The model under review builds one solid part; all positions refer to its coordinate system, in mm. A direction names the side the tool comes from. Coordinates: 2 decimals unless noted, no trailing zeros. Loops run counter-clockwise (first coordinate to the right, second up) from the corner with the lowest first, then second, coordinate; pieces in that order, holes last. Notation, with made-up numbers: (61.5, 70) - (83.5, 70) arc R15 ccw to (83.5, 74) - close; hole circle Ø9 at (63.25, 49). An arc over 180 degrees is marked (long way). Answer in a Markdown table with one row per item. Add a question column.
(1) We need section C-C on z = -5.25. Write out the cut boundary in (x, y), plus the area to 3 significant figures.
(2) We need section B-B on x = 0. Write out the cut boundary in (y, z), plus the area to 3 significant figures.
(3) Machinability: for faces 4 (the cylindrical face through (0.01, 55.65, -0.06)), 5 (the cylindrical face through (-0.867, 40.744, -4.93)), 6 (the flat face through (1, 48, -10)), which of the approach directions +Z, -Z, +X, -X, +Y, -Y give a long, thin tool a straight path to every point of the face, cutting with its end or side? Answer none if there is none.
(4) We need section A-A on y = 60.25. Write out the cut boundary in (x, z).
(5) For P1, Ø6, axis at y = 55.5, z = -4, coming from the -X side; P2, Ø2, axis at y = 52.5, z = -3, coming from the -X side; P3, Ø4, axis at y = 60.5, z = -0.5, coming from the +X side; P4, Ø3.5, axis at x = 0, y = 44.65, coming from the -Z side, all flat-tipped, find the tip position at first contact; note any pin that passes through.
(6) For line 1 along Y through (x, z) = (0, -6.3); line 2 along Y through (x, z) = (0.5, -6.75); line 3 along X through (y, z) = (62.25, -2.5), list the stretches that pass through material, from the lowest coordinate up.
(7) Mouldability with a two-part tool opening along X and no side actions: class faces 1 (the cylindrical face through (0.65, 41.72, -7.54)), 2 (the flat face through (2, 63.649, 0)), 3 (the cylindrical face through (0, 54, 4)) as +X half, -X half, draft (parallel to the pull), parting line (faces both ways), or undercut.
(8) We need section D-D on y = 51.25. Write out the cut boundary in (x, z).
from build123d import *

# Parameters (mm, degrees)
CROQUIS1_R              = 4
SALIENTE_EXTRUIR1_DEPTH = 10
CROQUIS3_R              = 3
CORTAR_EXTRUIR2_DEPTH   = 5
CROQUIS4_W              = 4
CROQUIS4_H              = 19
CROQUIS5_W              = 2
CROQUIS5_H              = 8


with BuildPart() as part:
    # Croquis1 → Saliente-Extruir1 (new body)
    with BuildSketch(Plane.XY):
        with Locations((0, 44.649122807)):
            Circle(CROQUIS1_R)
    extrude(amount=-SALIENTE_EXTRUIR1_DEPTH)

    # Croquis3 → Cortar-Extruir2 (cut)
    with BuildSketch(Plane(origin=(0, 0, -10), x_dir=(-1, 0, 0), z_dir=(0, 0, -1))):
        with Locations((0, 44.649122807)):
            Circle(CROQUIS3_R)
    extrude(amount=-CORTAR_EXTRUIR2_DEPTH, mode=Mode.SUBTRACT)

    # Croquis4 → Revolución1 (revolve)
    with BuildSketch(Plane(origin=(0, 0, 0), x_dir=(0, 0, -1), z_dir=(1, 0, 0)), mode=Mode.PRIVATE) as revoluci_n1_sk:
        with Locations((-2, 54.149122807)):
            Rectangle(CROQUIS4_W, CROQUIS4_H)
    revolve(revoluci_n1_sk.sketch.rotate(Axis((0, 44.649122807, 0), (0, 1, 0)), 180), axis=Axis((0, 44.649122807, 0), (0, 1, 0)))

    # Croquis5 → Cortar-Revolución1 (revolve, cut)
    with BuildSketch(Plane(origin=(0, 63.649122807, 0), x_dir=(1, 0, 0), z_dir=(0, 1, 0))):
        with Locations((0, 4)):
            Rectangle(CROQUIS5_W, CROQUIS5_H)
    revolve(axis=Axis((1, 63.649122807, 0), (-1, 0, 0)), mode=Mode.SUBTRACT)

    # Croquis6 → Revolución3 (revolve)
    with BuildSketch(Plane.XZ.offset(-44.649122807)):
        with BuildLine():
            Line((-4, 0), (4, 0))
            ThreePointArc((4, 0), (0, 4), (-4, 0))
        make_face()
    revolve(axis=Axis((-4, 44.649122807, 0), (1, 0, 0)))


solid = part.part
Outcome:
| question | item | result |
|---|---|---|
| 1 | outline | circle Ø8 at (0, 44.65); hole circle Ø6 at (0, 44.65) |
| 1 | area | 22.0 mm² |
| 2 | outline | (40.65, -10) - (41.65, -10) - (41.65, -5) - (47.65, -5) - (47.65, -10) - (48.65, -10) - (48.65, -4) - (56.72, -4) arc R8 cw to (56.72, 4) - (44.65, 4) arc R4 ccw to (40.65, 0) - close |
| 2 | area | 137 mm² |
| 3 | face 4 | +Y |
| 3 | face 5 | -Z |
| 3 | face 6 | -Z, +X, -X, +Y, -Y |
| 4 | outline | (-1, -3.87) - (-1, 3.87) arc R4 ccw to start; (1, -3.87) arc R4 ccw to (1, 3.87) - close |
| 5 | P1 | x = -3.87 |
| 5 | P2 | x = -3.46 |
| 5 | P3 | x = 4 |
| 5 | P4 | z = -5 |
| 6 | line 1 | 40.65 to 41.65, 47.65 to 48.65 |
| 6 | line 2 | 40.68 to 41.69, 47.61 to 48.62 |
| 6 | line 3 | -3.12 to -1, 1 to 3.12 |
| 7 | face 1 | undercut |
| 7 | face 2 | draft |
| 7 | face 3 | parting line |
| 8 | outline | circle Ø8 at (0, 0) |
